Check sheet for the modelled part. Datum: model origin and axes. Units: mm. Face numbers are marked on the shaded views. A direction names the side the tool comes from. Coordinates: 2 decimals unless noted, no trailing zeros. Write each loop counter-clockwise with the first axis right and the second up, starting at its lowest first coordinate (ties: lowest second). Pieces come first, ordered by that corner, then holes. Notation, with made-up numbers: (-3, 23) - (50, 23) arc R13 ccw to (50, 40) - close; hole circle Ø6 at (46, 65.5). An arc over 180 degrees is marked (long way). Use one line per item in the form item = value. Start each with the question number.
1. Go/stop test with flat-tipped pins: pin 1 Ø6 at (x, z) = (-4.5, -2) entering from -Y; pin 2 Ø12 at (y, z) = (19.5, -33.5) entering from +X. Record where each tip stops, or that it passes through.
2. Cross-section at A-A on y = 5.25. Record the boundary of the cut face in (x, z), then the cut area to 3 significant figures.
3. Tool access check on the marked faces 4 and 5. Record the directions out of +Z, -Z, +X, -X, +Y, -Y that give a thin tool (end or side, any length) a straight path to the whole face; none if there is none.
4. Cross-section at B-B on z = -20. Record the boundary of the cut face in (x, y).
5. Cross-section at D-D on z = 7. Record the boundary of the cut face in (x, y), then the cut area to 3 significant figures.
6. Cross-section at C-C on x = -1. Record the boundary of the cut face in (y, z), then the cut area to 3 significant figures.
7. Draft check along X on the marked faces 1, 2 and 3. Enter one of: +X half, -X half, draft (parallel to the pull), parting line (faces both ways), or undercut.
8. Scan lines: line 1 along X through (y, z) = (22.75, -13.5); line 2 along Z through (x, y) = (-9, 4.5); line 3 along Y through (x, z) = (5.5, 20.5). Record each from-to range of solid material in increasing order.
```python
from build123d import *

# Parameters (mm, degrees)
SKETCH2_W           = 68
SKETCH2_H           = 88
SKETCH2_W_2         = 62
SKETCH2_H_2         = 82
BOSS_EXTRUDE1_DEPTH = 30
CHAMFER1_SIZE       = 30
CHAMFER1_SIZE2      = 17.320508076
SHELL1_T            = -3
CUT_EXTRUDE1_REACH  = 77.039
SKETCH3_W           = 25.4
SKETCH3_H           = 25.4


with BuildPart() as part:
    # Sketch2 → Boss-Extrude1 (new body)
    # profile 1 of 2: a face of its own
    with BuildSketch(Plane(origin=(0, 0, 0), x_dir=(1, 0, 0), z_dir=(0, 1, 0))):
        Rectangle(SKETCH2_W, SKETCH2_H)
        Rectangle(SKETCH2_W_2, SKETCH2_H_2, mode=Mode.SUBTRACT)
    # profile 2 of 2: a face of its own
    with BuildSketch(Plane(origin=(0, 0, 0), x_dir=(1, 0, 0), z_dir=(0, 1, 0))):
        Rectangle(SKETCH2_W_2, SKETCH2_H_2)
    extrude(amount=BOSS_EXTRUDE1_DEPTH)

    # Chamfer1
    chamfer1_edges = [part.edges().sort_by_distance(p)[0] for p in [
        (0, 30, -44),
    ]]
    chamfer1_side = [part.faces().sort_by_distance(p)[0] for p in [
        (0, 30, 0),
    ]]
    chamfer(chamfer1_edges, length=CHAMFER1_SIZE, length2=CHAMFER1_SIZE2, reference=chamfer1_side[0])

    # Shell1
    shell1_openings = [part.faces().sort_by_distance(p)[0] for p in [
        (0, 0, 0),
    ]]
    offset(amount=SHELL1_T, openings=shell1_openings, kind=Kind.INTERSECTION)

    # Sketch3 → Cut-Extrude1 (cut, up to next)
    with BuildSketch(Plane(origin=(0, 28.562177826, -16.490381057), x_dir=(1, 0, 0), z_dir=(0, 0.8660254037844398, -0.4999999999999982)), mode=Mode.PRIVATE) as cut_extrude1_sk1:
        with Locations((0, 14.444863729)):
            Rectangle(SKETCH3_W, SKETCH3_H)
    cut_extrude1_tool1 = extrude(cut_extrude1_sk1.sketch, amount=-CUT_EXTRUDE1_REACH, mode=Mode.PRIVATE) & part.part
    add(cut_extrude1_tool1.solids().sort_by_distance((0, 21.339746, -29))[0], mode=Mode.SUBTRACT)


solid = part.part
```
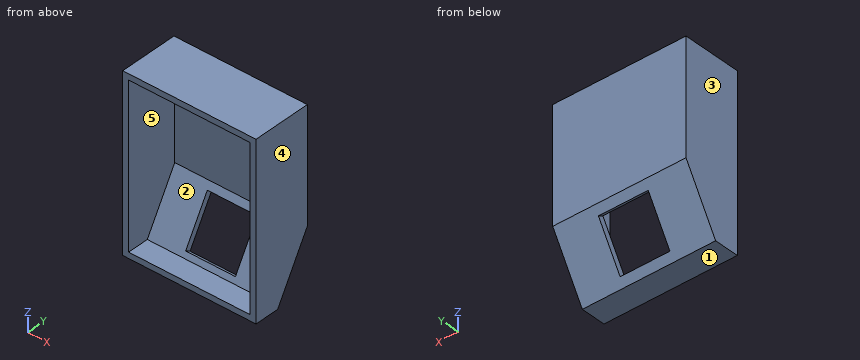
Final values:
q1.pin_1 = 27
q1.pin_2 = 34
q2.outline = (-34, -44) - (34, -44) - (34, 44) - (-34, 44) - close; hole (-31, -41) - (31, -41) - (31, 41) - (-31, 41) - close
q2.area = 900 mm²
q3.face_4 = +Z, -Z, +X, +Y, -Y
q3.face_5 = -Y
q4.outline = (-34, 0) - (-31, 0) - (-31, 23.07) - (-12.7, 23.07) - (-12.7, 26.54) - (-34, 26.54) - close; (12.7, 23.07) - (31, 23.07) - (31, 0) - (34, 0) - (34, 26.54) - (12.7, 26.54) - close
q5.outline = (-34, 0) - (-31, 0) - (-31, 27) - (31, 27) - (31, 0) - (34, 0) - (34, 30) - (-34, 30) - close
q5.area = 366 mm²
q6.outline = (0, -44) - (12.68, -44) - (14.99, -40) - (12.39, -38.5) - (10.95, -41) - (0, -41) - close; (0, 41) - (27, 41) - (27, -13.2) - (25.09, -16.5) - (27.69, -18) - (30, -14) - (30, 44) - (0, 44) - close
q6.area = 313 mm²
q7.face_1 = draft
q7.face_2 = undercut
q7.face_3 = -X half
q8.line_1 = -34 to -31, 31 to 34
q8.line_2 = -44 to -41, 41 to 44
q8.line_3 = 27 to 30
